Geometry check sheet. Reference: the model listing, model coordinates, mm. A direction names the side the tool comes from. Give positions to 0.01 mm unless a question says otherwise; leave off trailing zeros. Order: outer loops, then holes, each group sorted by start corner. A loop starts at its lowest first (then second) coordinate and runs counter-clockwise, first axis right, second up. Notation, with made-up numbers: M 38,20.25 L 80,20.25 A34 ccw 80,59.25 Z; hole C 84,10.5 d6. An arc over 180 degrees is marked long. Put each result on its own line as item: value. Start each with the question number.
Q1. Section check A-A on y = 0. Record the cut outline in (x, z), then the cut area to 3 significant figures.
Q2. Go/stop test with flat-tipped pins: pin 1 (4 mm diameter, centred on x = -3, z = 66, fed in from +Y); pin 2 (1.5 mm diameter, centred on y = 0.5, z = 42.5, fed in from +X); pin 3 (1 mm diameter, centred on x = 1, y = 4.5, fed in from -Z); pin 4 (3.5 mm diameter, centred on y = 0, z = 3.87, fed in from -X). Record where each tip stops, or that it passes through.
Q3. Section check B-B on y = -6. Record the cut outline in (x, z).
Q4. Material ranges on L1, parallel to Z at x = -1.1, y = 0; L2, parallel to Z at x = 2.25, y = 6.5; L3, parallel to Z at x = 1.25, y = 0.5, recorded low to high.
Q5. Access from +Z, -Z, +X, -X, +Y, -Y to the whole of each face (thin tool, end or side, straight path). Record for faces 1 (the flat face through (3.2, 1.8, 100)), 2 (the cylindrical face through (-7.493, 0.33, 109.86)).
Q6. Section check C-C on z = 16. Record the cut outline in (x, y), then the cut area to 3 significant figures.
```python
from build123d import *

# Parameters (mm, degrees)
SKETCH1_R               = 3.5
BOSS_EXTRUDE1_DEPTH     = 100
SKETCH2_R               = 7.5
BOSS_EXTRUDE2_DEPTH     = 20
SKETCH3_R               = 2
CUT_EXTRUDE1_DEPTH      = 8.5
CUT_EXTRUDE1_DEPTH_BACK = 8.5


with BuildPart() as part:
    # Sketch1 → Boss-Extrude1 (new body)
    with BuildSketch(Plane.XY):
        Circle(SKETCH1_R)
    extrude(amount=BOSS_EXTRUDE1_DEPTH)

    # Sketch2 → Boss-Extrude2 (add)
    with BuildSketch(Plane.XY.offset(100)):
        Circle(SKETCH2_R)
    extrude(amount=BOSS_EXTRUDE2_DEPTH)

    # Sketch3 → Cut-Extrude1 (cut, two sides)
    with BuildSketch(Plane(origin=(0, 0, 0), x_dir=(0, 0, -1), z_dir=(1, 0, 0))) as cut_extrude1_sk:
        with Locations((-3.868694711, 0)):
            Circle(SKETCH3_R)
    extrude(amount=CUT_EXTRUDE1_DEPTH, mode=Mode.SUBTRACT)
    extrude(cut_extrude1_sk.sketch, amount=-CUT_EXTRUDE1_DEPTH_BACK, mode=Mode.SUBTRACT)


solid = part.part
```
Results found:
1. outline: M -7.5,100 L -3.5,100 L -3.5,5.87 L 3.5,5.87 L 3.5,100 L 7.5,100 L 7.5,120 L -7.5,120 Z; M -3.5,0 L 3.5,0 L 3.5,1.87 L -3.5,1.87 Z
1. area: 972 mm^2
2. pin 1: stops at y = 3.35
2. pin 2: stops at x = 3.5
2. pin 3: stops at z = 100
2. pin 4: passes through
3. outline: M -4.5,100 L 4.5,100 L 4.5,120 L -4.5,120 Z
4. L1: z = 0 to 1.87, 5.87 to 120
4. L2: z = 100 to 120
4. L3: z = 0 to 1.93, 5.81 to 120
5. face 1: -Z
5. face 2: +Z, -Z
6. outline: C 0,0 d7
6. area: 38.5 mm^2
